For this review, take the finished solid that the model builds, in its own axes (mm). A direction names the side the tool comes from. Coordinates: 2 decimals unless noted, no trailing zeros. Loops run counter-clockwise (first coordinate to the right, second up) from the corner with the lowest first, then second, coordinate; pieces in that order, holes last. Notation, with made-up numbers: (41, -38.5) -> (77, -38.5) arc R30 ccw to (77, 0.5) -> close; hole circle Ø9 at (18.25, -30). An arc over 180 degrees is marked (long way). Answer in a Markdown table with one row per item.
from build123d import *

# Parameters (mm, degrees)
EXTRUDE_THIN1_DEPTH   = 100
IZIM1_R               = 3
KES_EKSTR_ZYON1_DEPTH = 20.32


with BuildPart() as part:
    # Sketch1 → Extrude-Thin1 (new body, symmetric)
    with BuildSketch(Plane.XY):
        with BuildLine():
            Line((-10, -7.5), (-10, 7.5))
            ThreePointArc((-10, 7.5), (-9.267766953, 9.267766953), (-7.5, 10))
            Line((-7.5, 10), (7.5, 10))
            ThreePointArc((7.5, 10), (9.267766953, 9.267766953), (10, 7.5))
            Line((10, 7.5), (10, -7.5))
            ThreePointArc((10, -7.5), (9.267766953, -9.267766953), (7.5, -10))
            Line((7.5, -10), (-7.5, -10))
            ThreePointArc((-7.5, -10), (-9.267766953, -9.267766953), (-10, -7.5))
        make_face()
        with BuildLine():
            Line((-8, -7.5), (-8, 7.5))
            ThreePointArc((-8, 7.5), (-7.853553391, 7.853553391), (-7.5, 8))
            Line((-7.5, 8), (7.5, 8))
            ThreePointArc((7.5, 8), (7.853553391, 7.853553391), (8, 7.5))
            Line((8, 7.5), (8, -7.5))
            ThreePointArc((8, -7.5), (7.853553391, -7.853553391), (7.5, -8))
            Line((7.5, -8), (-7.5, -8))
            ThreePointArc((-7.5, -8), (-7.853553391, -7.853553391), (-8, -7.5))
        make_face(mode=Mode.SUBTRACT)
    extrude(amount=EXTRUDE_THIN1_DEPTH, both=True)

    # Çizim1 → Kes-Ekstrüzyon1 (cut)
    with BuildSketch(Plane(origin=(10, 0, 0), x_dir=(0, 0, -1), z_dir=(1, 0, 0))):
        with Locations((80, 0)):
            Circle(IZIM1_R)
        with Locations((3.8, 0)):
            Circle(IZIM1_R)
    extrude(amount=-KES_EKSTR_ZYON1_DEPTH, mode=Mode.SUBTRACT)


solid = part.part
Item 1: Take a section at C-C, the plane x = 1. State the section outline as (y, z) points, and give its area (3 significant figures).
Worked answers:
| item | result |
|---|---|
| outline | (-10, -100) -> (-8, -100) -> (-8, 100) -> (-10, 100) -> close; (8, -100) -> (10, -100) -> (10, 100) -> (8, 100) -> close |
| area | 800 mm² |
Item 2: For L1, parallel to X at y = -6.5, z = -43; L2, parallel to Y at x = -9.2, z = -3.8, list the stretches that pass through material, from the lowest coordinate up.
Worked answers:
| item | result |
|---|---|
| L1 | -10 to -8, 8 to 10 |
| L2 | -9.33 to -3, 3 to 9.33 |
Item 3: Take a section at D-D, the plane z = -9. State the section outline as (x, y) points, and give its area (3 significant figures).
Worked answers:
| item | result |
|---|---|
| outline | (-10, -7.5) arc R2.5 ccw to (-7.5, -10) -> (7.5, -10) arc R2.5 ccw to (10, -7.5) -> (10, 7.5) arc R2.5 ccw to (7.5, 10) -> (-7.5, 10) arc R2.5 ccw to (-10, 7.5) -> close; hole (-8, -7.5) arc R0.5 ccw to (-7.5, -8) -> (7.5, -8) arc R0.5 ccw to (8, -7.5) -> (8, 7.5) arc R0.5 ccw to (7.5, 8) -> (-7.5, 8) arc R0.5 ccw to (-8, 7.5) -> close |
| area | 139 mm² |
Item 4: The part is to be moulded in two halves that separate along Y. For faces 3 (the cylindrical face through (9.014, -2.662, -5.184)), 4 (the flat face through (10, 0, 1)), 5 (the flat face through (0, 10, 1)), say which applies: +Y half, -Y half, draft (parallel to the pull), parting line (faces both ways), or undercut.
Worked answers:
| item | result |
|---|---|
| face 3 | undercut |
| face 4 | draft |
| face 5 | +Y half |
Item 5: For faces 1 (the cylindrical face through (-8.986, -2.662, -5.184)), 2 (the flat face through (0, -8, 1)), list the 3-axis set-ups (+Z, -Z, +X, -X, +Y, -Y) from which the entire face can be reached by the end or side of a thin tool; tool diameter is ignored.
Worked answers:
| item | result |
|---|---|
| face 1 | +X, -X |
| face 2 | +Z, -Z |
Item 6: Take a section at A-A, the plane y = 0. State the section outline as (x, z) points.
Worked answers:
| item | result |
|---|---|
| outline | (-10, -100) -> (-8, -100) -> (-8, -83) -> (-10, -83) -> close; (-10, -77) -> (-8, -77) -> (-8, -6.8) -> (-10, -6.8) -> close; (-10, -0.8) -> (-8, -0.8) -> (-8, 100) -> (-10, 100) -> close; (8, -100) -> (10, -100) -> (10, -83) -> (8, -83) -> close; (8, -77) -> (10, -77) -> (10, -6.8) -> (8, -6.8) -> close; (8, -0.8) -> (10, -0.8) -> (10, 100) -> (8, 100) -> close |
Item 7: Take a section at B-B, the plane z = -80. State the section outline as (x, y) points, and give its area (3 significant figures).
Worked answers:
| item | result |
|---|---|
| outline | (-10, -7.5) arc R2.5 ccw to (-7.5, -10) -> (7.5, -10) arc R2.5 ccw to (10, -7.5) -> (10, -3) -> (8, -3) -> (8, -7.5) arc R0.5 cw to (7.5, -8) -> (-7.5, -8) arc R0.5 cw to (-8, -7.5) -> (-8, -3) -> (-10, -3) -> close; (-10, 3) -> (-8, 3) -> (-8, 7.5) arc R0.5 cw to (-7.5, 8) -> (7.5, 8) arc R0.5 cw to (8, 7.5) -> (8, 3) -> (10, 3) -> (10, 7.5) arc R2.5 ccw to (7.5, 10) -> (-7.5, 10) arc R2.5 ccw to (-10, 7.5) -> close |
| area | 115 mm² |
